The listing builds one solid part. Answer for the finished solid, in the listing's coordinates (mm). A direction names the side the tool comes from. Coordinates: 2 decimals unless noted, no trailing zeros. Loops run counter-clockwise (first coordinate to the right, second up) from the corner with the lowest first, then second, coordinate; pieces in that order, holes last. Notation, with made-up numbers: (81.5, 1) -> (112.5, 1) arc R27 cw to (112.5, 31) -> close; hole circle Ø6 at (45.5, 47.25). An arc over 180 degrees is marked (long way). Answer in a Markdown table with one row per item.
```python
from build123d import *

# Parameters (mm, degrees)
F0_W     = 210
F0_H     = 125
F1_DEPTH = 6.4
F3_DEPTH = 25
F5_DEPTH = 6.4
F6_SIZE  = 10
F7_W     = 69
F7_H     = 95
F8_DEPTH = 6.401
F9_SIZE  = 10


with BuildPart() as f1:
    # F0 (on Top) → F1 (new body)
    with BuildSketch(Plane.XY):
        Rectangle(F0_W, F0_H)
    extrude(amount=F1_DEPTH)

    # F2 (on face) → F3 (cut)
    with BuildSketch(Plane.XY.offset(6.4)):
        Polygon((105, 16.5), (56, 16.5), (50.90122, 15.692433), (46.301543, 13.34878), (42.65122, 9.698457), (40.307567, 5.09878), (39.5, 0), (40.307567, -5.09878), (42.65122, -9.698457), (46.301543, -13.34878), (50.90122, -15.692433), (56, -16.5), (105, -16.5), align=None)
    extrude(amount=-F3_DEPTH, mode=Mode.SUBTRACT)

    # F4 (on Top) → F5 (cut, through all)
    with BuildSketch(Plane.XY):
        Polygon((94.661921, 53.473939), (95, 53.37467), (95.338079, 53.473939), (95.56882, 53.740228), (95.618965, 54.088994), (95.472593, 54.409504), (95.176176, 54.6), (94.823824, 54.6), (94.527407, 54.409504), (94.381035, 54.088994), (94.43118, 53.740228), align=None)
        Polygon((95.472593, -54.409504), (95.618965, -54.088994), (95.56882, -53.740228), (95.338079, -53.473939), (95, -53.37467), (94.661921, -53.473939), (94.43118, -53.740228), (94.381035, -54.088994), (94.527407, -54.409504), (94.823824, -54.6), (95.176176, -54.6), align=None)
        Polygon((23.37082, 53.48961), (23.6, 53.805048), (23.6, 54.194952), (23.37082, 54.51039), (23, 54.630877), (22.62918, 54.51039), (22.4, 54.194952), (22.4, 53.805048), (22.62918, 53.48961), (23, 53.369123), align=None)
        Polygon((22.62918, -53.48961), (22.4, -53.805048), (22.4, -54.194952), (22.62918, -54.51039), (23, -54.630877), (23.37082, -54.51039), (23.6, -54.194952), (23.6, -53.805048), (23.37082, -53.48961), (23, -53.369123), align=None)
    extrude(amount=F5_DEPTH, mode=Mode.SUBTRACT)

    # F6
    f6_edges = [f1.edges().sort_by_distance(p)[0] for p in [
        (-105, 62.5, 3.2),
        (105, 62.5, 3.2),
        (105, -62.5, 3.2),
        (-105, -62.5, 3.2),
    ]]
    chamfer(f6_edges, length=F6_SIZE)

    # F7 (on face) → F8 (cut, through all)
    with BuildSketch(Plane(origin=(0, 0, 0), x_dir=(1, 0, 0), z_dir=(0, 0, -1))):
        with Locations((-50.5, 0)):
            Rectangle(F7_W, F7_H)
    extrude(amount=-F8_DEPTH, mode=Mode.SUBTRACT)

    # F9
    f9_edges = [f1.edges().sort_by_distance(p)[0] for p in [
        (-85, 47.5, 3.2),
        (-16, 47.5, 3.2),
        (-16, -47.5, 3.2),
        (-85, -47.5, 3.2),
    ]]
    chamfer(f9_edges, length=F9_SIZE)


solid = f1.part
```
Item 1: A cutting plane is placed at A-A, the plane x = -47. Determine the outline of the cut face in (y, z), plus the area to 3 significant figures.
Findings below:
| item | result |
|---|---|
| outline | (-62.5, 0) -> (-47.5, 0) -> (-47.5, 6.4) -> (-62.5, 6.4) -> close; (47.5, 0) -> (62.5, 0) -> (62.5, 6.4) -> (47.5, 6.4) -> close |
| area | 192 mm2 |
Item 2: A cutting plane is placed at B-B, the plane y = 41. Determine the outline of the cut face in (x, z), plus the area to 3 significant figures.
Findings below:
| item | result |
|---|---|
| outline | (-105, 0) -> (-81.5, 0) -> (-81.5, 6.4) -> (-105, 6.4) -> close; (-19.5, 0) -> (105, 0) -> (105, 6.4) -> (-19.5, 6.4) -> close |
| area | 947 mm2 |
Item 3: Flat-ended cylindrical pins translate along their axes: pin 1 Ø2 at (y, z) = (2.5, 2) entering from +X; pin 2 Ø1 at (x, y) = (-7, 45.5) entering from -Z. Find the tip coordinate at first contact, or state that the pin passes through.
Findings below:
| item | result |
|---|---|
| pin 1 | stops at x = 40.05 |
| pin 2 | stops at z = 0 |
Item 4: A tool of negligible diameter and unlimited length cuts with its end or side. For faces 1 (the face through (-16, 1, 3)), 2 (the face through (48.569, -14.504, 3.245)), 3 (the face through (-1, -62.5, 3)), from which of +Z, -Z, +X, -X, +Y, -Y can it reach the whole face along a straight path? Write none if from no direction.
Findings below:
| item | result |
|---|---|
| face 1 | +Z, -Z |
| face 2 | +Z, -Z, +X |
| face 3 | +Z, -Z, +X, -X, -Y |
Item 5: A cutting plane is placed at C-C, the plane z = 3.75. Count the separate pieces of the cut face and the enclosed holes in it, plus the area to 3 significant figures.
Findings below:
| item | result |
|---|---|
| separate pieces | 1 |
| enclosed holes | 5 |
| area | 17,700 mm2 |
Item 6: Find the intervals of material crossed by probe 1 along X at (y, z) = (23.5, 5.25); probe 2 along Y at (x, z) = (-68.5, 2); probe 3 along Y at (x, z) = (87, 1.25), in increasing order.
Findings below:
| item | result |
|---|---|
| probe 1 | x = -105 to -85, -16 to 105 |
| probe 2 | y = -62.5 to -47.5, 47.5 to 62.5 |
| probe 3 | y = -62.5 to -16.5, 16.5 to 62.5 |
Item 7: Determine the mould class of faces 4 (the face through (100.1, 57.4, 3.2)), 5 (the face through (41.496, 7.431, 3.245)), 6 (the face through (-99.9, -57.6, 3.2)) for opening direction Y: +Y half, -Y half, draft (parallel to the pull), parting line (faces both ways), or undercut.
Findings below:
| item | result |
|---|---|
| face 4 | +Y half |
| face 5 | undercut |
| face 6 | -Y half |
